Verification items for the finished model (mm, model axes). Face numbers are marked on the shaded views. A direction names the side the tool comes from. Give positions to 0.01 mm unless a question says otherwise; leave off trailing zeros. Loops run counter-clockwise (first coordinate to the right, second up) from the corner with the lowest first, then second, coordinate; pieces in that order, holes last. Notation, with made-up numbers: M 64.5,63.25 L 93.5,63.25 A22 cw 93.5,88.25 Z; hole C 80.5,-5.5 d6. An arc over 180 degrees is marked long. Answer in a Markdown table with one row per item.
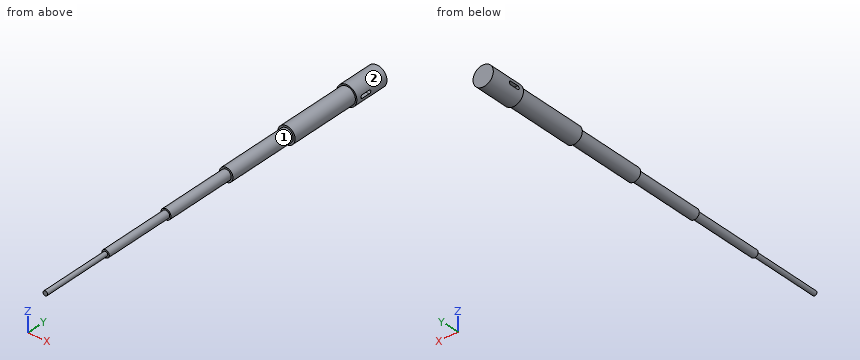
```python
from build123d import *

# Parameters (mm, degrees)
F0_R      = 1.387608
F1_DEPTH  = 5
F2_R      = 1.189862
F3_DEPTH  = 10
F4_R      = 0.933138
F5_DEPTH  = 10
F6_R      = 0.70066
F7_DEPTH  = 10
F8_R      = 0.509978
F9_DEPTH  = 10
F10_R     = 0.309305
F11_DEPTH = 10
F13_DEPTH = 12.5


with BuildPart() as f1:
    # F0 (on Front) → F1 (new body)
    with BuildSketch(Plane.XZ):
        Circle(F0_R)
    extrude(amount=F1_DEPTH)

    # F2 (on face) → F3 (join)
    with BuildSketch(Plane.XZ.offset(5)):
        Circle(F2_R)
    extrude(amount=F3_DEPTH)

    # F4 (on face) → F5 (join)
    with BuildSketch(Plane.XZ.offset(15)):
        Circle(F4_R)
    extrude(amount=F5_DEPTH)

    # F6 (on face) → F7 (join)
    with BuildSketch(Plane.XZ.offset(25)):
        Circle(F6_R)
    extrude(amount=F7_DEPTH)

    # F8 (on face) → F9 (join)
    with BuildSketch(Plane.XZ.offset(35)):
        Circle(F8_R)
    extrude(amount=F9_DEPTH)

    # F10 (on face) → F11 (join)
    with BuildSketch(Plane.XZ.offset(45)):
        Circle(F10_R)
    extrude(amount=F11_DEPTH)

    # F12 (on Right) → F13 (cut, symmetric)
    with BuildSketch(Plane.YZ):
        with BuildLine():
            Line((-2.909436, 0.232579), (-4.072334, 0.232579))
            ThreePointArc((-4.072334, 0.232579), (-4.304913, 0), (-4.072334, -0.232579))
            Line((-4.072334, -0.232579), (-2.909436, -0.232579))
            ThreePointArc((-2.909436, -0.232579), (-2.676857, 0), (-2.909436, 0.232579))
        make_face()
    extrude(amount=F13_DEPTH, both=True, mode=Mode.SUBTRACT)


solid = f1.part
```
Item 1: Scan lines: L1, parallel to Y at x = -0.7, z = 0.55; L2, parallel to Z at x = -0.4, y = -39; L3, parallel to Y at x = -0.2, z = 0.15. Record each from-to range of solid material in increasing order. Write a range as [from, to].
Reported:
| item | result |
|---|---|
| L1 | y = [-25, 0] |
| L2 | z = [-0.32, 0.32] |
| L3 | y = [-55, -4.25], [-2.73, 0] |
Item 2: Sectioned sample at A-A (y = -46). Record the cut outline in (x, z).
Reported:
| item | result |
|---|---|
| outline | C 0,0 d0.62 |
Item 3: Tool access check on the marked faces 1 and 2. Record the directions out of +Z, -Z, +X, -X, +Y, -Y that give a thin tool (end or side, any length) a straight path to the whole face; none if there is none.
Reported:
| item | result |
|---|---|
| face 1 | -Y |
| face 2 | +Y, -Y |
Item 4: Go/stop test with flat-tipped pins: pin 1 (1.5 mm diameter, centred on y = -39.5, z = -0.5, fed in from +X); pin 2 (1.5 mm diameter, centred on x = 1, y = -19, fed in from -Z). Record where each tip stops, or that it passes through.
Reported:
| item | result |
|---|---|
| pin 1 | stops at x = 0.51 |
| pin 2 | stops at z = -0.9 |
Item 5: Sectioned sample at B-B (y = -36). Record the cut outline in (x, z).
Reported:
| item | result |
|---|---|
| outline | C 0,0 d1.02 |
